Verification items for this drawing (mm, ordinates from the low corner). Round coordinates to 2 decimals unless told otherwise and drop trailing zeros. Order: outer loops, then holes, each group sorted by start corner. A loop starts at its lowest first (then second) coordinate and runs counter-clockwise, first axis right, second up. Notation, with made-up numbers: (-24, -33.75) - (20, -33.75) arc R7 cw to (20, -26.75) - close; hole circle Ø10 at (-29.5, -13). An arc over 180 degrees is marked (long way). Return JSON: item names as keys, results as strings. Group by question number.
Q1. Sectioned sample at A-A, the plane y = 21. Record the cut outline in (x, z), then the cut area to 4 significant figures.
Q2. Sectioned sample at C-C, the plane x = 35.5. Record the cut outline in (y, z), then the cut area to 3 significant figures.
Q3. Material ranges on line 1 along X through (y, z) = (8, 14.5) (1 decimal); line 2 along X through (y, z) = (17, 12.25); line 3 along Y through (x, z) = (33.5, 4.75), recorded low to high.
Q4. Gauge pin test, flat ends, axial feed: pin 1 Ø10 at (x, z) = (42.5, 22) entering from -Y; pin 2 Ø1 at (x, y) = (37, 13.5) entering from +Z; pin 3 Ø3 at (x, y) = (16, 31) entering from -Z; pin 4 Ø5 at (y, z) = (5, 15.5) entering from +X. Record the tip position at first contact, or that the pin passes through.
Q5. Sectioned sample at D-D, the plane z = 2.5. Record the cut outline in (x, y).
Q6. Sectioned sample at B-B, the plane z = 23.5. Record the cut outline in (x, y).
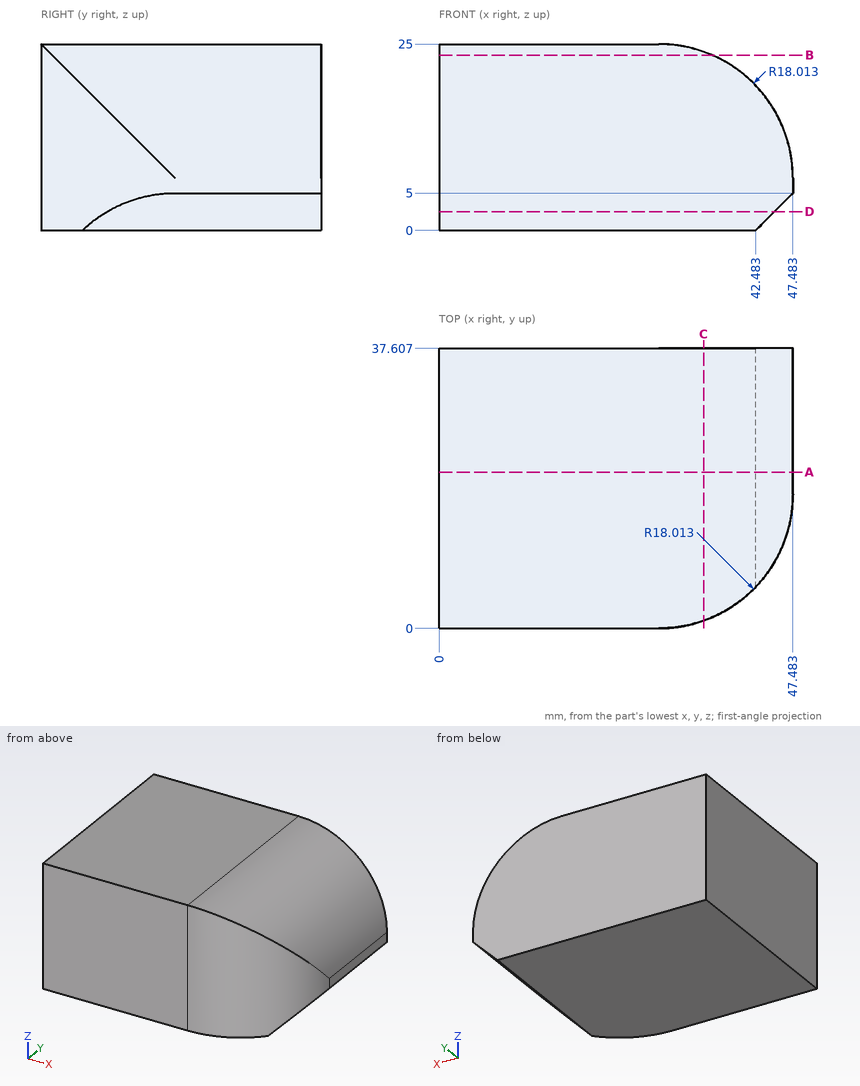
Reply:
{
 "1": {"outline": "(0, 0) - (42.48, 0) - (47.48, 5) - (47.48, 6.99) arc R18.01 ccw to (29.47, 25) - (0, 25) - close", "area": "1,105 mm^2"},
 "2": {"outline": "(1.04, 0) - (37.61, 0) - (37.61, 23.96) - (1.04, 23.96) - close", "area": "876 mm^2"},
 "3": {"line 1": "0 to 44.4", "line 2": "0 to 46.7", "line 3": "0.46 to 37.61"},
 "4": {"pin 1": "y = 1.89", "pin 2": "z = 23.57", "pin 3": "z = 0", "pin 4": "x = 44.1"},
 "5": {"outline": "(0, 0) - (29.47, 0) arc R18.01 ccw to (44.98, 8.86) - (44.98, 37.61) - (0, 37.61) - close"},
 "6": {"outline": "(0, 0) - (29.47, 0) arc R18.01 ccw to (36.67, 1.5) - (36.67, 37.61) - (0, 37.61) - close"}
}
